Build history of the part. All positions in model axes, mm. A direction names the side the tool comes from. Round coordinates to 2 decimals unless told otherwise and drop trailing zeros. Write each loop counter-clockwise with the first axis right and the second up, starting at its lowest first coordinate (ties: lowest second). Pieces come first, ordered by that corner, then holes. Notation, with made-up numbers: M -11.75,29 L 1.25,29 A23 ccw 1.25,64 Z; hole C 56,-21.75 d9. An arc over 180 degrees is marked long. Write item = value, one per line. Start each with the question number.
Q1. Band-saw the part on C-C on z = -61. Write the cut outline in (x, y), plus the area to 3 significant figures.
Q2. Band-saw the part on B-B on x = -63. Write the cut outline in (y, z), plus the area to 3 significant figures.
Q3. Tool access for faces 4 (the flat face through (-61.56, 1.48, -22.98)), 5 (the flat face through (-16, 1, -30)), 6 (the flat face through (-12.75, 1, 2)), 7 (the flat face through (-29.98, 1.48, -4.44)), 8 (the flat face through (-43.02, 1.48, -54.56)): list every direction of +Z, -Z, +X, -X, +Y, -Y with a clear straight run to the whole face (end or side of a thin tool).
Q4. Drop flat-ended pins along their axis: P1, Ø3, axis at x = -49.5, z = -29.5, coming from the +Y side; P2, Ø1.8, axis at x = -36.5, z = -16.5, coming from the -Y side; P3, Ø0.9, axis at x = -37.5, y = 2, coming from the -Z side. Give the stop position or say it passes through.
Q5. Pull direction Z, two halves, no side cores. Call faces 1 (the flat face through (-60.25, 1, 2)), 2 (the flat face through (-37, 1, -50)), 3 (the flat face through (-36, 3, -30)): released by +Z, released by -Z, zero draft, split by the parting line, or undercut.
Q6. Band-saw the part on A-A on z = -10. Write the cut outline in (x, y), plus the area to 3 significant figures.
Q7. Band-saw the part on D-D on x = -36.5. Write the cut outline in (y, z).
Q8. Probe L1, parallel to X at y = 2.35, z = -60; L2, parallel to X at y = 1.1, z = -42.5; L3, parallel to X at y = 1.85, z = -29.5. List the from-to ranges inside material, lowest first.
```python
from build123d import *

# Parameters (mm, degrees)
SKETCH1_R           = 1
SKETCH1_W           = 3
SKETCH1_H           = 10
SKETCH1_W_2         = 10
SKETCH1_H_2         = 3
BOSS_EXTRUDE1_DEPTH = 3


with BuildPart() as part:
    # Sketch1 → Boss-Extrude1 (new body)
    with BuildSketch(Plane(origin=(0, 0, 0), x_dir=(1, 0, 0), z_dir=(0, 1, 0))):
        Polygon((-31.5, 9), (-41.5, 9), (-44.5, 0), (-44.5, -7), (-73, -7), (-73, 21.5), (-66, 21.5), (-57, 24.5), (-57, 34.5), (-66, 37.5), (-73, 37.5), (-73, 66), (-44.5, 66), (-44.5, 59), (-41.5, 50), (-31.5, 50), (-28.5, 59), (-28.5, 66), (0, 66), (0, 37.5), (-7, 37.5), (-16, 34.5), (-16, 24.5), (-7, 21.5), (0, 21.5), (0, -7), (-28.5, -7), (-28.5, 0), align=None)
        with Locations(Location((-36.5, 42.5, 0), (0, 0, 270))):
            Circle(SKETCH1_R, mode=Mode.SUBTRACT)
        with Locations(Location((-23.5, 29.5, 0), (0, 0, 270))):
            Circle(SKETCH1_R, mode=Mode.SUBTRACT)
        with Locations(Location((-36.5, 16.5, 0), (0, 0, 270))):
            Circle(SKETCH1_R, mode=Mode.SUBTRACT)
        with Locations(Location((-49.5, 29.5, 0), (0, 0, 270))):
            Circle(SKETCH1_R, mode=Mode.SUBTRACT)
        with Locations((-5.5, 48.25)):
            Rectangle(SKETCH1_W, SKETCH1_H, mode=Mode.SUBTRACT)
        with Locations((-5.5, 10.75)):
            Rectangle(SKETCH1_W, SKETCH1_H, mode=Mode.SUBTRACT)
        with Locations((-67.5, 10.75)):
            Rectangle(SKETCH1_W, SKETCH1_H, mode=Mode.SUBTRACT)
        with Locations((-67.5, 48.25)):
            Rectangle(SKETCH1_W, SKETCH1_H, mode=Mode.SUBTRACT)
        with Locations((-55.25, -1.5)):
            Rectangle(SKETCH1_W_2, SKETCH1_H_2, mode=Mode.SUBTRACT)
        with Locations((-17.75, -1.5)):
            Rectangle(SKETCH1_W_2, SKETCH1_H_2, mode=Mode.SUBTRACT)
        with Locations((-17.75, 60.5)):
            Rectangle(SKETCH1_W_2, SKETCH1_H_2, mode=Mode.SUBTRACT)
        with Locations((-55.25, 60.5)):
            Rectangle(SKETCH1_W_2, SKETCH1_H_2, mode=Mode.SUBTRACT)
    extrude(amount=BOSS_EXTRUDE1_DEPTH)


solid = part.part
```
Conclusion:
q1.outline = M -73,0 L -60.25,0 L -60.25,3 L -73,3 Z; M -50.25,0 L -44.5,0 L -44.5,3 L -50.25,3 Z; M -28.5,0 L -22.75,0 L -22.75,3 L -28.5,3 Z; M -12.75,0 L 0,0 L 0,3 L -12.75,3 Z
q1.area = 111 mm^2
q2.outline = M 0,-66 L 3,-66 L 3,-36.5 L 0,-36.5 Z; M 0,-22.5 L 3,-22.5 L 3,7 L 0,7 Z
q2.area = 177 mm^2
q3.face_4 = -X, +Y, -Y
q3.face_5 = +X, +Y, -Y
q3.face_6 = +Y, -Y
q3.face_7 = +Z, +Y, -Y
q3.face_8 = -Z, +Y, -Y
q4.P1 = 3
q4.P2 = through
q4.P3 = -50
q5.face_1 = undercut
q5.face_2 = released by -Z
q5.face_3 = zero draft
q6.outline = M -73,0 L -69,0 L -69,3 L -73,3 Z; M -66,0 L -7,0 L -7,3 L -66,3 Z; M -4,0 L 0,0 L 0,3 L -4,3 Z
q6.area = 201 mm^2
q7.outline = M 0,-50 L 3,-50 L 3,-43.5 L 0,-43.5 Z; M 0,-41.5 L 3,-41.5 L 3,-17.5 L 0,-17.5 Z; M 0,-15.5 L 3,-15.5 L 3,-9 L 0,-9 Z
q8.L1 = -73 to -60.25, -50.25 to -44.5, -28.5 to -22.75, -12.75 to 0
q8.L2 = -73 to -37.5, -35.5 to 0
q8.L3 = -57 to -50.5, -48.5 to -24.5, -22.5 to -16
